Read the model definition and answer for the solid it produces. Units are mm, in the model's axes. A direction names the side the tool comes from. Coordinates: 2 decimals unless noted, no trailing zeros. Loops run counter-clockwise (first coordinate to the right, second up) from the corner with the lowest first, then second, coordinate; pieces in that order, holes last. Notation, with made-up numbers: M 87,35.5 L 145,35.5 A17 cw 145,56.5 Z; hole C 72.5,-15 d9. An arc over 180 degrees is marked long. One line per item, written item: value. Start each with the question number.
1. For faces 4 (the face through (3, 0.5, 4.5)), 5 (the face through (6.5, 0, 4.5)), 6 (the face through (1.5, 0.5, 4)), 7 (the face through (2, 6, 4)), determine the directions among +Z, -Z, +X, -X, +Y, -Y from which every point of the face is accessible in a straight line to the end or side of a thin tool.
2. The part is cut by section C-C (y = 2.25). Write down the section's boundary in (x, z).
3. The part is cut by section A-A (z = 0.4). Write down the section's boundary in (x, y), then the cut area to 3 significant figures.
4. The part is cut by section B-B (x = 5.25). Write down the section's boundary in (y, z), then the cut area to 3 significant figures.
5. Flat-ended cylindrical pins translate along their axes: pin 1 (2 mm diameter, centred on y = 5, z = 1, fed in from -X); pin 2 (0.5 mm diameter, centred on y = 7, z = 4.5, fed in from -X); pin 3 (0.6 mm diameter, centred on x = 6, z = 2.5, fed in from -Y); pin 4 (2 mm diameter, centred on x = 1, z = 3.5, fed in from +Y). Find the tip coordinate at first contact, or state that the pin passes through.
6. Determine the mould class of faces 1 (the face through (1.9, 6.14, 2.99)), 2 (the face through (3, 0.5, 1)), 3 (the face through (1, 0, 1)) for opening direction X: +X half, -X half, draft (parallel to the pull), parting line (faces both ways), or undercut.
7. Consider probe 1 along Y at (x, z) = (4, 0.5); probe 2 along X at (y, z) = (4, 1.4); probe 3 along X at (y, z) = (0.5, 1.55). Determine where each line is inside the solid, lowest interval first.
8. The part is cut by section D-D (z = 4.6). Write down the section's boundary in (x, y), then the cut area to 3 significant figures.
```python
from build123d import *

# Parameters (mm, degrees)
SKETCH2_R           = 2
BOSS_EXTRUDE1_DEPTH = 2
BOSS_EXTRUDE2_DEPTH = 2
SKETCH4_W           = 3
SKETCH4_H           = 1.003544002
BOSS_EXTRUDE3_DEPTH = 1


with BuildPart() as part:
    # Sketch2 → Boss-Extrude1 (new body)
    with BuildSketch(Plane.XY):
        with BuildLine():
            Line((0, 0), (3, 0))
            Line((3, 0), (3, 1))
            Line((3, 1), (5, 1))
            Line((5, 1), (5, 0))
            Line((5, 0), (8, 0))
            Line((8, 0), (8, 4))
            ThreePointArc((8, 4), (4, 8), (0, 4))
            Line((0, 4), (0, 0))
        make_face()
        with Locations((4, 4)):
            Circle(SKETCH2_R, mode=Mode.SUBTRACT)
    extrude(amount=BOSS_EXTRUDE1_DEPTH)

    # Sketch3 → Boss-Extrude2 (add)
    with BuildSketch(Plane.XY.offset(2)):
        with BuildLine():
            Line((4, 8), (4, 7))
            ThreePointArc((4, 7), (1.878679656, 6.121320344), (1, 4))
            Line((1, 4), (0, 4))
            Line((0, 4), (0, 1.003544002))
            Line((0, 1.003544002), (8, 1.003544002))
            Line((8, 1.003544002), (8, 4))
            ThreePointArc((8, 4), (6.828427125, 6.828427125), (4, 8))
        make_face()
        with BuildLine():
            ThreePointArc((6, 4), (4, 2), (2, 4))
            ThreePointArc((2, 4), (2.585786438, 5.414213562), (4, 6))
            ThreePointArc((4, 6), (5.414213562, 5.414213562), (6, 4))
        make_face(mode=Mode.SUBTRACT)
    extrude(amount=BOSS_EXTRUDE2_DEPTH)

    # Sketch4 → Boss-Extrude3 (add)
    with BuildSketch(Plane.XY.offset(4)):
        with BuildLine():
            Line((1, 4), (0, 4))
            Line((0, 4), (0, 1.003544002))
            Line((0, 1.003544002), (3, 1.003544002))
            Line((3, 1.003544002), (8, 1.003544002))
            Line((8, 1.003544002), (8, 4))
            ThreePointArc((8, 4), (6.828427125, 6.828427125), (4, 8))
            Line((4, 8), (4, 7))
            Line((4, 7), (4, 6))
            ThreePointArc((4, 6), (5.414213562, 5.414213562), (6, 4))
            ThreePointArc((6, 4), (4, 2), (2, 4))
            Line((2, 4), (1, 4))
        make_face()
        with Locations((1.5, 0.501772001)):
            Rectangle(SKETCH4_W, SKETCH4_H)
        Polygon((8, 1.003544002), (3, 1.003544002), (5, 1), (5, 0), (8, 0), align=None)
    extrude(amount=BOSS_EXTRUDE3_DEPTH)


solid = part.part
```
Answer block:
1. face 4: +Z, -Z, -Y
1. face 5: +Z, -Z, +X, -X, -Y
1. face 6: +X, -X, -Y
1. face 7: +Z, -X, +Y
2. outline: M 0,0 L 3.03,0 L 3.03,5 L 0,5 Z; M 4.97,0 L 8,0 L 8,5 L 4.97,5 Z
3. outline: M 0,0 L 3,0 L 3,1 L 5,1 L 5,0 L 8,0 L 8,4 A4 ccw 0,4 Z; hole C 4,4 d4
3. area: 42.6 mm2
4. outline: M 0,0 L 2.44,0 L 2.44,5 L 0,5 L 0,4 L 1,4 L 1,2 L 0,2 Z; M 5.56,0 L 7.8,0 L 7.8,5 L 5.56,5 Z
4. area: 21.4 mm2
5. pin 1: stops at x = 0
5. pin 2: stops at x = 4
5. pin 3: stops at y = 1
5. pin 4: stops at y = 6.24
6. face 1: -X half
6. face 2: undercut
6. face 3: draft
7. probe 1: y = 1 to 2, 6 to 8
7. probe 2: x = 0 to 2, 6 to 8
7. probe 3: x = 0 to 3, 5 to 8
8. outline: M 0,0 L 3,0 L 3,1 L 5,1 L 5,0 L 8,0 L 8,4 A4 ccw 4,8 L 4,6 A2 cw long 2,4 L 0,4 Z
8. area: 33.1 mm2
